from build123d import *

# Parameters (mm, degrees)
BOSS_EXTRUDE1_DEPTH = 12
FILLET4_R           = 1
FILLET5_R           = 2
FILLET6_R           = 2
CUT_EXTRUDE3_DEPTH  = 33
FILLET8_R           = 2
BOSS_EXTRUDE2_DEPTH = 12
FILLET9_R           = 1
FILLET10_R          = 1
BOSS_EXTRUDE3_DEPTH = 12
FILLET11_R          = 2
FILLET12_R          = 1
FILLET13_R          = 2
SKETCH10_R          = 2.5
CUT_EXTRUDE4_DEPTH  = 18


with BuildPart() as part:
    # Sketch2 → Boss-Extrude1 (new body)
    with BuildSketch(Plane(origin=(0, 0, 0), x_dir=(1, 0, 0), z_dir=(0, 1, 0))):
        with BuildLine():
            Line((0, 0), (-0.73121606, 5.95527691))
            ThreePointArc((-0.73121606, 5.95527691), (15.138799382, 10.254914459), (31.320769044, 13.168354193))
            Line((31.320769044, 13.168354193), (30.087748344, 23.210501924))
            ThreePointArc((30.087748344, 23.210501924), (94.266191099, 25.160742626), (157.417218543, 13.557997867))
            ThreePointArc((157.417218543, 13.557997867), (158.923283556, 4.547467734), (151, 0))
            ThreePointArc((151, 0), (75.5, 10), (0, 0))
        make_face()
    extrude(amount=BOSS_EXTRUDE1_DEPTH)

    # Fillet4
    fillet4_edges = [part.edges().sort_by_distance(p)[0] for p in [
        (30.087748344, 6, -23.210501924),
    ]]
    fillet(fillet4_edges, radius=FILLET4_R)

    # Fillet5
    fillet5_edges = [part.edges().sort_by_distance(p)[0] for p in [
        (31.320769044, 6, -13.168354193),
    ]]
    fillet(fillet5_edges, radius=FILLET5_R)

    # Fillet6
    fillet6_edges = [part.edges().sort_by_distance(p)[0] for p in [
        (-0.73121606, 6, -5.95527691),
    ]]
    fillet(fillet6_edges, radius=FILLET6_R)

    # Sketch5 → Cut-Extrude3 (cut)
    with BuildSketch(Plane(origin=(0, 0, 0), x_dir=(1, 0, 0), z_dir=(0, 1, 0))):
        with BuildLine():
            Line((35.656168792, 18.886901985), (36.452121023, 12.404391276))
            ThreePointArc((36.452121023, 12.404391276), (94.477597701, 14.388970685), (151.768043541, 4.970939327))
            ThreePointArc((151.768043541, 4.970939327), (153.480302105, 5.560994433), (154.540953062, 7.028991016))
            ThreePointArc((154.540953062, 7.028991016), (154.409459032, 8.592099199), (153.190642938, 9.579563223))
            ThreePointArc((153.190642938, 9.579563223), (94.887793134, 20.097584909), (35.656168792, 18.886901985))
        make_face()
    extrude(amount=CUT_EXTRUDE3_DEPTH, mode=Mode.SUBTRACT)

    # Fillet8
    fillet8_edges = [part.edges().sort_by_distance(p)[0] for p in [
        (35.656168792, 6, -18.886901985),
        (36.452121023, 6, -12.404391276),
    ]]
    fillet(fillet8_edges, radius=FILLET8_R)

    # Sketch6 → Boss-Extrude2 (add)
    with BuildSketch(Plane(origin=(0, 0, 0), x_dir=(1, 0, 0), z_dir=(0, 1, 0))):
        with BuildLine():
            Line((0, 0), (0.243738687, -1.985092303))
            ThreePointArc((0.243738687, -1.985092303), (9.813572193, 0.430074334), (19.460534614, 2.515945677))
            Line((19.460534614, 2.515945677), (20.460534614, 4.729325881))
            ThreePointArc((20.460534614, 4.729325881), (10.187446562, 2.549918803), (0, 0))
        make_face()
    extrude(amount=BOSS_EXTRUDE2_DEPTH)

    # Fillet9
    fillet9_edges = [part.edges().sort_by_distance(p)[0] for p in [
        (0.243738687, 6, 1.985092303),
    ]]
    fillet(fillet9_edges, radius=FILLET9_R)

    # Fillet10
    fillet10_edges = [part.edges().sort_by_distance(p)[0] for p in [
        (20.460534614, 6, -4.729325881),
        (19.460534614, 6, -2.515945677),
    ]]
    fillet(fillet10_edges, radius=FILLET10_R)

    # Sketch7 → Boss-Extrude3 (add)
    with BuildSketch(Plane(origin=(0, 0, 0), x_dir=(1, 0, 0), z_dir=(0, 1, 0))):
        with BuildLine():
            Line((70, 9.947842385), (74, 7.996093893))
            ThreePointArc((74, 7.996093893), (81.502036249, 7.937453494), (89, 7.683433507))
            Line((89, 7.683433507), (92, 9.530243228))
            ThreePointArc((92, 9.530243228), (81.003961961, 9.947767207), (70, 9.947842385))
        make_face()
    extrude(amount=BOSS_EXTRUDE3_DEPTH)

    # Fillet11
    fillet11_edges = [part.edges().sort_by_distance(p)[0] for p in [
        (70, 6, -9.947842385),
    ]]
    fillet(fillet11_edges, radius=FILLET11_R)

    # Fillet12
    fillet12_edges = [part.edges().sort_by_distance(p)[0] for p in [
        (74, 6, -7.996093893),
        (89, 6, -7.683433507),
    ]]
    fillet(fillet12_edges, radius=FILLET12_R)

    # Fillet13
    fillet13_edges = [part.edges().sort_by_distance(p)[0] for p in [
        (92, 6, -9.530243228),
    ]]
    fillet(fillet13_edges, radius=FILLET13_R)

    # Sketch10 → Cut-Extrude4 (cut)
    with BuildSketch(Plane.XY):
        with Locations((81.692531177, 6)):
            Circle(SKETCH10_R)
        with Locations((10.103466275, 6)):
            Circle(SKETCH10_R)
    extrude(amount=-CUT_EXTRUDE4_DEPTH, mode=Mode.SUBTRACT)


solid = part.part
Check sheet for the modelled part. Datum: model origin and axes. Units: mm. A direction names the side the tool comes from. Give positions to 0.01 mm unless a question says otherwise; leave off trailing zeros. Loops run counter-clockwise (first coordinate to the right, second up) from the corner with the lowest first, then second, coordinate; pieces in that order, holes last. Notation, with made-up numbers: M -37.75,56.25 L -11.75,56.25 A28 ccw -11.75,78.25 Z; hole C 30.5,-21.5 d10. An arc over 180 degrees is marked long. Use a Markdown table: item, result. Add a question column.
Q1. Tool access check on faces 1 (the cylindrical face through (94.681, 5.916, -14.376)), 2 (the cylindrical face through (45.476, 5.916, -8.442)), 3 (the flat face through (30.65, 5.92, -18.62)). Record the directions out of +Z, -Z, +X, -X, +Y, -Y that give a thin tool (end or side, any length) a straight path to the whole face; none if there is none.
Q2. Go/stop test with flat-tipped pins: pin 1 (6.5 mm diameter, centred on x = 10.1, y = 6, fed in from +Z); pin 2 (3 mm diameter, centred on x = 142, z = -10.5, fed in from -Y); pin 3 (4 mm diameter, centred on x = 81.69, y = 6, fed in from +Z); pin 4 (2 mm diameter, centred on x = 31, y = 8, fed in from -Z). Record where each tip stops, or that it passes through.
Q3. Scan lines: line 1 along Z through (x, y) = (73, 5.25); line 2 along Y through (x, z) = (82, -11); line 3 along Z through (x, y) = (120, 3.75). Record each from-to range of solid material in increasing order. Write a range as [from, to].
Q4. Sectioned sample at B-B, the plane x = 26. Record the cut outline in (y, z), then the cut area to 3 significant figures.
Q5. Sectioned sample at A-A, the plane x = 111. Record the cut outline in (y, z).
Q6. Mould release check, pull along Z, two halves, no side actions. Record for faces 4 (the cylindrical face through (9.78, 8.48, -4.77)), 5 (the cylindrical face through (153.46, 5.916, -5.546)), 6 (the cylindrical face through (158.98, 5.92, -4.67)): pulls with the +Z half, pulls with the -Z half, needs draft (parallel to the pull), parting line crosses it, or undercut.
Verdict:
| question | item | result |
|---|---|---|
| 1 | face 1 | +Y, -Y |
| 1 | face 2 | +Z, +Y, -Y |
| 1 | face 3 | -X, +Y, -Y |
| 2 | pin 1 | z = 0.28 |
| 2 | pin 2 | through |
| 2 | pin 3 | z = -20.77 |
| 2 | pin 4 | z = -23.47 |
| 3 | line 1 | [-26.02, -21.02], [-14.99, -8.48] |
| 3 | line 2 | [0, 3.52], [8.48, 12] |
| 3 | line 3 | [-22.1, -17.03], [-11.62, -6.57] |
| 4 | outline | M 0,-12.37 L 12,-12.37 L 12,-5.74 L 0,-5.74 Z |
| 4 | area | 79.5 mm^2 |
| 5 | outline | M 0,-23.42 L 12,-23.42 L 12,-18.38 L 0,-18.38 Z; M 0,-12.86 L 12,-12.86 L 12,-7.82 L 0,-7.82 Z |
| 6 | face 4 | needs draft |
| 6 | face 5 | undercut |
| 6 | face 6 | parting line crosses it |
